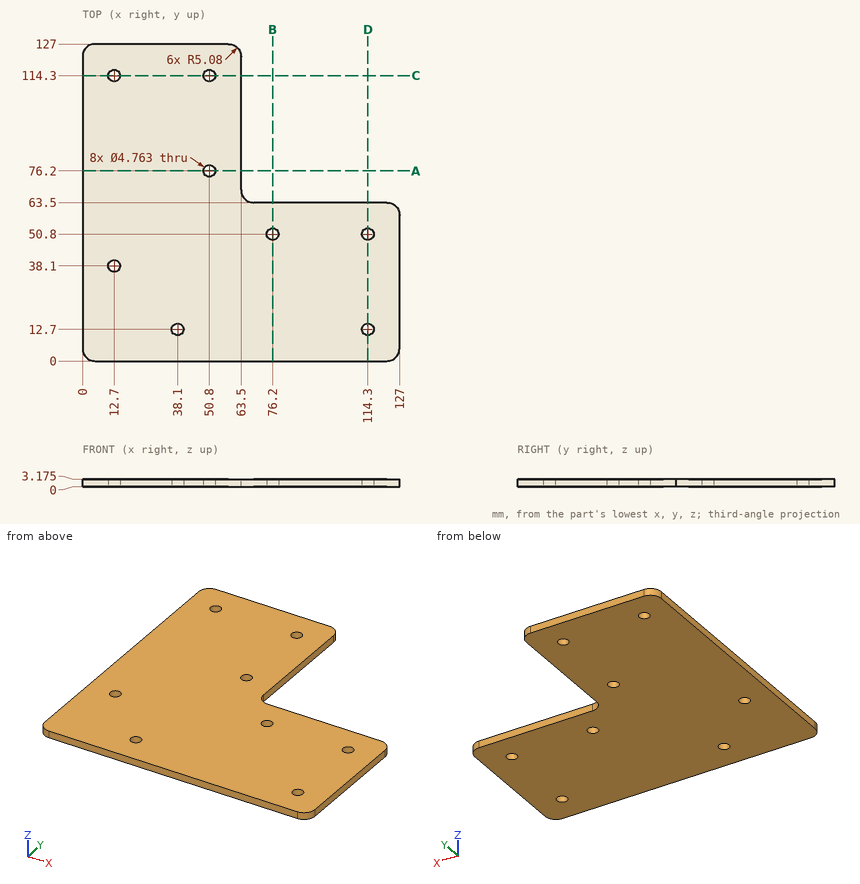
For this review, use the dimensioned drawing (mm, ordinates from the lowest corner) and the shaded views. Round coordinates to 2 decimals unless told otherwise and drop trailing zeros. Write each loop counter-clockwise with the first axis right and the second up, starting at its lowest first coordinate (ties: lowest second). Pieces come first, ordered by that corner, then holes. Notation, with made-up numbers: (-15, 74) - (24, 74) arc R13 cw to (24, 90) - close; hole circle Ø2 at (18, -37). An arc over 180 degrees is marked (long way). Answer as a JSON object with one key per item and string values.
1. To check wall thickness, follow line 1 along Y through (x, z) = (12.7, 1.2); line 2 along X through (y, z) = (76.5, 2.75); line 3 along X through (y, z) = (114.5, 0.3). State the ranges of each line that lie inside material, in increasing order.
Response values:
{"line 1": "y = 0 to 35.72, 40.48 to 111.92, 116.68 to 127", "line 2": "x = 0 to 48.44, 53.16 to 63.5", "line 3": "x = 0 to 10.33, 15.07 to 48.43, 53.17 to 63.5"}
2. For pin 1 Ø1.5 at (x, z) = (67.5, 2) entering from +Y; pin 2 Ø1 at (y, z) = (105.5, 1.5) entering from -X; pin 3 Ø1.5 at (x, z) = (91.5, 1.5) entering from +Y, all flat-tipped, find the tip position at first contact; note any pin that passes through.
Response values:
{"pin 1": "stops at y = 63.84", "pin 2": "stops at x = 0", "pin 3": "stops at y = 63.5"}
3. We need section A-A on y = 76.2. Give the boundary of the cut face in (x, z) (1 decimal).
Response values:
{"outline": "(0, 0) - (48.4, 0) - (48.4, 3.2) - (0, 3.2) - close; (53.2, 0) - (63.5, 0) - (63.5, 3.2) - (53.2, 3.2) - close"}
4. We need section C-C on y = 114.3. Give the boundary of the cut face in (x, z) (1 decimal), then the cut area to 3 significant figures.
Response values:
{"outline": "(0, 0) - (10.3, 0) - (10.3, 3.2) - (0, 3.2) - close; (15.1, 0) - (48.4, 0) - (48.4, 3.2) - (15.1, 3.2) - close; (53.2, 0) - (63.5, 0) - (63.5, 3.2) - (53.2, 3.2) - close", "area": "171 mm2"}
